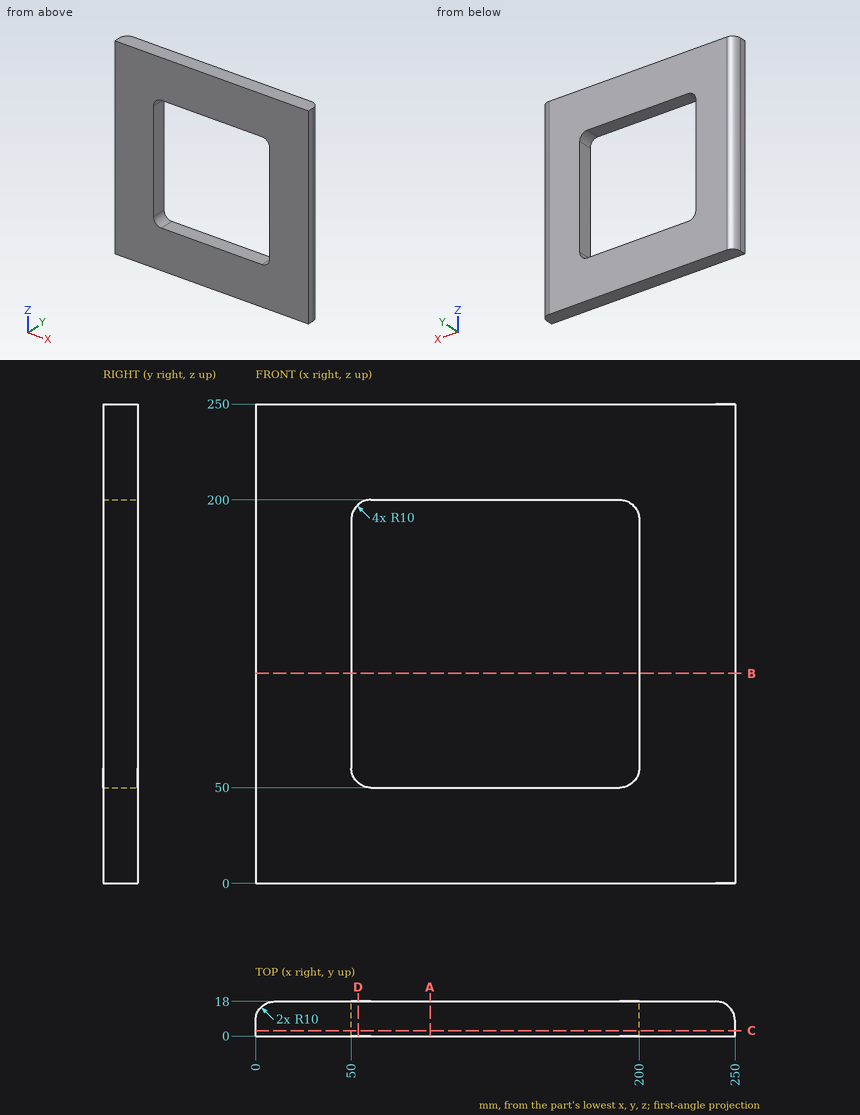
Drawing for the job (mm, zero at the part's lowest x, y, z). Round coordinates to 2 decimals unless told otherwise and drop trailing zeros. Loops run counter-clockwise (first coordinate to the right, second up) from the corner with the lowest first, then second, coordinate; pieces in that order, holes last. Notation, with made-up numbers: (24, 26.5) -> (82, 26.5) arc R22 ccw to (82, 42.5) -> close; hole circle Ø3 at (0.5, -31.5). An arc over 180 degrees is marked (long way). Answer in a Markdown table with one row per item.
Item 1: Drill centre lines: L1, parallel to X at y = 5.5, z = 85; L2, parallel to X at y = 1.75, z = 57. Where is each one in solid material? Low to high. Write a range as [from, to].
Answers below:
| item | result |
|---|---|
| L1 | x = [0, 50], [200, 250] |
| L2 | x = [0, 50.46], [199.54, 250] |
Item 2: Saw through at A-A (x = 91). Write the cut outline in (y, z), and give its area (3 significant figures).
Answers below:
| item | result |
|---|---|
| outline | (0, 0) -> (18, 0) -> (18, 50) -> (0, 50) -> close; (0, 200) -> (18, 200) -> (18, 250) -> (0, 250) -> close |
| area | 1,800 mm² |
Item 3: Pin check, flat tips, straight feed: pin 1 (5 mm diameter, centred on x = 152, y = 12, fed in from -Z); pin 2 (1 mm diameter, centred on y = 10, z = 121.5, fed in from -X). Stop position of each tip, or through.
Answers below:
| item | result |
|---|---|
| pin 1 | stops at z = 0 |
| pin 2 | stops at x = 0.11 |
Item 4: Saw through at D-D (x = 53.5). Write the cut outline in (y, z).
Answers below:
| item | result |
|---|---|
| outline | (0, 0) -> (18, 0) -> (18, 52.4) -> (0, 52.4) -> close; (0, 197.6) -> (18, 197.6) -> (18, 250) -> (0, 250) -> close |
Item 5: Saw through at B-B (z = 109.5). Write the cut outline in (x, y), and give its area (3 significant figures).
Answers below:
| item | result |
|---|---|
| outline | (0, 0) -> (50, 0) -> (50, 18) -> (10, 18) arc R10 ccw to (0, 8) -> close; (200, 0) -> (250, 0) -> (250, 8) arc R10 ccw to (240, 18) -> (200, 18) -> close |
| area | 1,760 mm² |
Item 6: Saw through at C-C (y = 2.75). Write the cut outline in (x, z), and give its area (3 significant figures).
Answers below:
| item | result |
|---|---|
| outline | (0, 0) -> (250, 0) -> (250, 250) -> (0, 250) -> close; hole (50, 60) arc R10 ccw to (60, 50) -> (190, 50) arc R10 ccw to (200, 60) -> (200, 190) arc R10 ccw to (190, 200) -> (60, 200) arc R10 ccw to (50, 190) -> close |
| area | 40,100 mm² |
